Could you check a few things on this model? Use its own coordinates, in mm. Give positions to 0.01 mm unless a question says otherwise; leave off trailing zeros. Write each loop counter-clockwise with the first axis right and the second up, starting at its lowest first coordinate (ties: lowest second). Pieces come first, ordered by that corner, then holes. Notation, with made-up numbers: M -3.75,27 L 39.25,27 A22 ccw 39.25,49 Z; hole C -21,-30 d11. An arc over 180 degrees is marked long. Use one line per item in the form item = value.
from build123d import *

# Parameters (mm, degrees)
SKETCH6_W           = 286.5
SKETCH6_H           = 115
BOSS_EXTRUDE3_DEPTH = 5
SKETCH7_R           = 2.5
CUT_EXTRUDE1_DEPTH  = 13
SKETCH8_R           = 125
CUT_EXTRUDE4_DEPTH  = 10


with BuildPart() as part:
    # Sketch6 → Boss-Extrude3 (new body)
    with BuildSketch(Plane.XY):
        with Locations((18.25, 57.5)):
            Rectangle(SKETCH6_W, SKETCH6_H)
    extrude(amount=BOSS_EXTRUDE3_DEPTH)

    # Sketch7 → Cut-Extrude1 (cut)
    with BuildSketch(Plane.XY.offset(5)):
        with Locations((151.1, 111)):
            Circle(SKETCH7_R)
        with Locations((126.1, 111)):
            Circle(SKETCH7_R)
        with Locations((-114.6, 111)):
            Circle(SKETCH7_R)
        with Locations((-89.6, 111)):
            Circle(SKETCH7_R)
    extrude(amount=-CUT_EXTRUDE1_DEPTH, mode=Mode.SUBTRACT)

    # Sketch8 → Cut-Extrude4 (cut)
    with BuildSketch(Plane.XY.offset(5)):
        with Locations((18.25, -80)):
            Circle(SKETCH8_R)
    extrude(amount=-CUT_EXTRUDE4_DEPTH, mode=Mode.SUBTRACT)


solid = part.part
1) I want a section at D-D, the plane y = 16. Please give me the cut outline in (x, z).
Checked values:
outline = M -125,0 L -61.81,0 L -61.81,5 L -125,5 Z; M 98.31,0 L 161.5,0 L 161.5,5 L 98.31,5 Z
2) Thinking about a two-plate mould opening in X: for faces 1 (the cylindrical face through (19.78, 44.99, 2.54)), 2 (the flat face through (-102, 0, 2)), 3 (the flat face through (161.5, 57, 2)), 4 (the flat face through (-125, 57, 2)), which applies, released by +X, released by -X, zero draft, split by the parting line, or undercut?
Checked values:
face_1 = undercut
face_2 = zero draft
face_3 = released by +X
face_4 = released by -X
3) I want a section at B-B, the plane x = 151.1. Please give me the cut outline in (y, z), plus the area to 3 significant figures.
Checked values:
outline = M 0,0 L 108.5,0 L 108.5,5 L 0,5 Z; M 113.5,0 L 115,0 L 115,5 L 113.5,5 Z
area = 550 mm2
4) I want a section at C-C, the plane z = 3. Please give me the cut outline in (x, y), plus the area to 3 significant figures.
Checked values:
outline = M -125,0 L -77.8,0 A125 cw 114.3,0 L 161.5,0 L 161.5,115 L -125,115 Z; hole C -114.6,111 d5; hole C -89.6,111 d5; hole C 126.1,111 d5; hole C 151.1,111 d5
area = 26,900 mm2
5) I want a section at A-A, the plane y = 111. Please give me the cut outline in (x, z), plus the area to 3 significant figures.
Checked values:
outline = M -125,0 L -117.1,0 L -117.1,5 L -125,5 Z; M -112.1,0 L -92.1,0 L -92.1,5 L -112.1,5 Z; M -87.1,0 L 123.6,0 L 123.6,5 L -87.1,5 Z; M 128.6,0 L 148.6,0 L 148.6,5 L 128.6,5 Z; M 153.6,0 L 161.5,0 L 161.5,5 L 153.6,5 Z
area = 1,330 mm2
6) For pin 1 Ø3 at (x, z) = (11.5, 1) entering from -Y; pin 2 Ø1 at (x, z) = (13, 3) entering from -Y, each with a flat end and sliding along its axis, tell me the tip position at first contact or that it passes through.
Checked values:
pin_1 = 44.73
pin_2 = 44.87
7) If I drill on L1, parallel to Y at x = -89.6, z = 1.55; L2, parallel to X at y = 31, z = 3.95; L3, parallel to X at y = 26, z = 4.4, over which ranges is the centre line in solid material (lowest first)?
Checked values:
L1 = 0 to 108.5, 113.5 to 115
L2 = -125 to -39.23, 75.73 to 161.5
L3 = -125 to -48, 84.5 to 161.5
